Can you work these out from the model? Positions are in its coordinate system, mm. A direction names the side the tool comes from. Give positions to 0.01 mm unless a question says otherwise; leave off trailing zeros. Loops run counter-clockwise (first coordinate to the right, second up) from the corner with the lowest first, then second, coordinate; pieces in that order, holes last. Notation, with made-up numbers: (42, -35.75) - (65, -35.75) arc R24 ccw to (65, -15.75) - close; hole circle Ø6 at (38.5, -14). An arc over 180 degrees is marked (long way). Answer as a JSON object with one key per item and string values.
```python
from build123d import *

# Parameters (mm, degrees)
SKETCH1_W                                   = 304.8
SKETCH1_H                                   = 76.2
BOSS_EXTRUDE1_DEPTH                         = 6.35
SKETCH3_W                                   = 25.4
SKETCH3_H                                   = 50.8
CUT_EXTRUDE2_DEPTH                          = 25.4
BOSS_EXTRUDE2_DEPTH                         = 19.05
BOSS_EXTRUDE3_DEPTH                         = 304.8
BOSS_EXTRUDE4_DEPTH                         = 15.24
BOSS_EXTRUDE5_DEPTH                         = 15.24
CBORE_FOR_8_BINDING_HEAD_MACHINE_SC_2_COUNT = 2
CBORE_FOR_8_BINDING_HEAD_MACHINE_SC_2_PITCH = 238.76
CBORE_FOR_8_BINDING_HEAD_MACHINE_SC_3_COUNT = 2
CBORE_FOR_8_BINDING_HEAD_MACHINE_SC_3_PITCH = 255.670904094
CBORE_FOR_8_BINDING_HEAD_MACHINE_SC_4_COUNT = 2
CBORE_FOR_8_BINDING_HEAD_MACHINE_SC_4_PITCH = 91.44
SKETCH12_R                                  = 2.2479
CUT_EXTRUDE3_DEPTH                          = 23.0345001


with BuildPart() as part:
    # Sketch1 → Boss-Extrude1 (new body)
    with BuildSketch(Plane(origin=(0, 0, 0), x_dir=(1, 0, 0), z_dir=(0, 1, 0))):
        Rectangle(SKETCH1_W, SKETCH1_H)
    extrude(amount=-BOSS_EXTRUDE1_DEPTH)

    # Sketch3 → Cut-Extrude2 (cut)
    with BuildSketch(Plane(origin=(0, 0, 0), x_dir=(1, 0, 0), z_dir=(0, 1, 0))):
        with Locations((133.35, 0)):
            Rectangle(SKETCH3_W, SKETCH3_H)
    extrude(amount=-CUT_EXTRUDE2_DEPTH, mode=Mode.SUBTRACT)

    # Sketch4 → Boss-Extrude2 (add)
    with BuildSketch(Plane(origin=(0, 0, 0), x_dir=(1, 0, 0), z_dir=(0, 1, 0))):
        Polygon((152.4, 38.1), (-152.4, 38.1), (-152.4, 31.75), (146.05, 31.75), (152.4, 31.75), align=None)
        Polygon((146.05, -31.75), (-152.4, -31.75), (-152.4, -38.1), (152.4, -38.1), (152.4, -31.75), align=None)
        Polygon((152.4, -31.75), (152.4, 31.75), (146.05, 31.75), (146.05, 25.4), (146.05, -25.4), (146.05, -31.75), align=None)
    extrude(amount=BOSS_EXTRUDE2_DEPTH)

    # Sketch5 → Boss-Extrude3 (add)
    with BuildSketch(Plane.ZY.offset(152.4)):
        with BuildLine():
            Line((38.1, -6.35), (-38.1, -6.35))
            Line((-38.1, -6.35), (-38.1, -12.7))
            ThreePointArc((-38.1, -12.7), (0, -25.4), (38.1, -12.7))
            Line((38.1, -12.7), (38.1, -6.35))
        make_face()
    extrude(amount=-BOSS_EXTRUDE3_DEPTH)

    # Sketch8 → Boss-Extrude4 (add)
    with BuildSketch(Plane.ZY.offset(127)):
        with BuildLine():
            Line((-38.1, -12.7), (-38.1, 6.6675))
            Line((-38.1, 6.6675), (-53.34, 6.6675))
            Line((-53.34, 6.6675), (-53.34, 3.645763686))
            ThreePointArc((-53.34, 3.645763686), (-46.444745641, -5.202835962), (-38.1, -12.7))
        make_face()
        with BuildLine():
            Line((53.34, 3.645763686), (53.34, 6.6675))
            Line((53.34, 6.6675), (38.1, 6.6675))
            Line((38.1, 6.6675), (38.1, -12.7))
            ThreePointArc((38.1, -12.7), (46.444745641, -5.202835962), (53.34, 3.645763686))
        make_face()
    extrude(amount=-BOSS_EXTRUDE4_DEPTH)

    # Sketch9 → Boss-Extrude5 (add)
    with BuildSketch(Plane.ZY.offset(-111.76)):
        with BuildLine():
            Line((-38.1, -12.7), (-38.1, 6.6675))
            Line((-38.1, 6.6675), (-53.34, 6.6675))
            Line((-53.34, 6.6675), (-53.34, 3.645763686))
            ThreePointArc((-53.34, 3.645763686), (-46.444745641, -5.202835962), (-38.1, -12.7))
        make_face()
        with BuildLine():
            Line((53.34, 3.645763686), (53.34, 6.6675))
            Line((53.34, 6.6675), (38.1, 6.6675))
            Line((38.1, 6.6675), (38.1, -12.7))
            ThreePointArc((38.1, -12.7), (46.444745641, -5.202835962), (53.34, 3.645763686))
        make_face()
    extrude(amount=-BOSS_EXTRUDE5_DEPTH)

    # Sketch11 → CBORE for #8 Binding Head Machine Screw1 (revolve, cut)
    with BuildSketch(Plane(origin=(-119.38, -6.0325, -45.72), x_dir=(0, 0, -1), z_dir=(1, 0, 0))):
        Polygon((0, 0), (0, 25.0825), (2.2479, 25.0825), (2.2479, 2.667), (4.7625, 2.667), (4.7625, 0), align=None)
    cbore_for_8_binding_head_machine_screw1 = revolve(axis=Axis((-119.38, -12.3825, -45.72), (0, 1, 0)), mode=Mode.SUBTRACT)

    # CBORE for _8 Binding Head Machine Sc 2: CBORE for #8 Binding Head Machine Screw1 ×2
    with Locations(*[(i * CBORE_FOR_8_BINDING_HEAD_MACHINE_SC_2_PITCH, 0, 0) for i in range(1, CBORE_FOR_8_BINDING_HEAD_MACHINE_SC_2_COUNT)]):
        add(cbore_for_8_binding_head_machine_screw1, mode=Mode.SUBTRACT)

    # CBORE for _8 Binding Head Machine Sc 3: CBORE for #8 Binding Head Machine Screw1 ×2
    with Locations(*[Vector(0.933856752, 0, 0.357647267) * (i * CBORE_FOR_8_BINDING_HEAD_MACHINE_SC_3_PITCH) for i in range(1, CBORE_FOR_8_BINDING_HEAD_MACHINE_SC_3_COUNT)]):
        add(cbore_for_8_binding_head_machine_screw1, mode=Mode.SUBTRACT)

    # CBORE for _8 Binding Head Machine Sc 4: CBORE for #8 Binding Head Machine Screw1 ×2
    with Locations(*[(0, 0, i * CBORE_FOR_8_BINDING_HEAD_MACHINE_SC_4_PITCH) for i in range(1, CBORE_FOR_8_BINDING_HEAD_MACHINE_SC_4_COUNT)]):
        add(cbore_for_8_binding_head_machine_screw1, mode=Mode.SUBTRACT)

    # Sketch12 → Cut-Extrude3 (cut, through all)
    with BuildSketch(Plane.XZ.offset(3.3655)):
        with BuildLine():
            Line((-123.509642203, -48.092227124), (-115.250357797, -48.092227124))
            ThreePointArc((-115.250357797, -48.092227124), (-119.38, -40.9575), (-123.509642203, -48.092227124))
        make_face()
        with BuildLine():
            ThreePointArc((-114.6175, -45.72), (-120.607596281, -41.118433569), (-123.509642203, -48.092227124))
            Line((-123.509642203, -48.092227124), (-115.250357797, -48.092227124))
            ThreePointArc((-115.250357797, -48.092227124), (-114.778433569, -46.947596281), (-114.6175, -45.72))
        make_face()
        with BuildLine():
            Line((-115.250357797, -48.092227124), (-123.509642203, -48.092227124))
            ThreePointArc((-123.509642203, -48.092227124), (-119.38, -50.4825), (-115.250357797, -48.092227124))
        make_face()
        with BuildLine():
            Line((-123.509642203, 48.092227124), (-115.250357797, 48.092227124))
            ThreePointArc((-115.250357797, 48.092227124), (-119.38, 50.4825), (-123.509642203, 48.092227124))
        make_face()
        with BuildLine():
            ThreePointArc((-123.509642203, 48.092227124), (-119.38, 40.9575), (-115.250357797, 48.092227124))
            Line((-115.250357797, 48.092227124), (-123.509642203, 48.092227124))
        make_face()
        with Locations((-119.38, 45.72)):
            Circle(SKETCH12_R, mode=Mode.SUBTRACT)
        with BuildLine():
            ThreePointArc((124.1425, 45.72), (123.981566431, 46.947596281), (123.509642203, 48.092227124))
            Line((123.509642203, 48.092227124), (115.250357797, 48.092227124))
            ThreePointArc((115.250357797, 48.092227124), (118.152403719, 41.118433569), (124.1425, 45.72))
        make_face()
        with BuildLine():
            Line((115.250357797, 48.092227124), (123.509642203, 48.092227124))
            ThreePointArc((123.509642203, 48.092227124), (119.38, 50.4825), (115.250357797, 48.092227124))
        make_face()
        with BuildLine():
            Line((123.509642203, 48.092227124), (115.250357797, 48.092227124))
            ThreePointArc((115.250357797, 48.092227124), (119.38, 40.9575), (123.509642203, 48.092227124))
        make_face()
        with BuildLine():
            Line((115.250357797, -48.092227124), (123.509642203, -48.092227124))
            ThreePointArc((123.509642203, -48.092227124), (119.38, -40.9575), (115.250357797, -48.092227124))
        make_face()
        with BuildLine():
            ThreePointArc((124.1425, -45.72), (118.152403719, -41.118433569), (115.250357797, -48.092227124))
            Line((115.250357797, -48.092227124), (123.509642203, -48.092227124))
            ThreePointArc((123.509642203, -48.092227124), (123.981566431, -46.947596281), (124.1425, -45.72))
        make_face()
        with BuildLine():
            Line((123.509642203, -48.092227124), (115.250357797, -48.092227124))
            ThreePointArc((115.250357797, -48.092227124), (119.38, -50.4825), (123.509642203, -48.092227124))
        make_face()
        with Locations((-119.38, 45.72)):
            Circle(SKETCH12_R)
    extrude(amount=CUT_EXTRUDE3_DEPTH, mode=Mode.SUBTRACT)


solid = part.part
```
1) Imagine slicing it at A-A on x = -19. Write out the boundary of the cut face in (y, z).
Check sheet entries:
{"outline": "(-12.7, -38.1) - (19.05, -38.1) - (19.05, -31.75) - (0, -31.75) - (0, 31.75) - (19.05, 31.75) - (19.05, 38.1) - (-12.7, 38.1) arc R63.5 ccw to start"}
2) I need wall thicknesses on L1, parallel to X at y = 2.25, z = -45.72; L2, parallel to X at y = -5.3, z = 45.72; L3, parallel to Z at x = 46, y = 1. Which ranges of each line are inside material? Lowest first, please.
Check sheet entries:
{"L1": "-127 to -121.63, -117.13 to -111.76, 111.76 to 117.13, 121.63 to 127", "L2": "-127 to -124.14, -114.62 to -111.76, 111.76 to 114.62, 124.14 to 127", "L3": "-38.1 to -31.75, 31.75 to 38.1"}
3) Imagine slicing it at D-D on y = -16. Write out the boundary of the cut face in (x, z).
Check sheet entries:
{"outline": "(-152.4, -33.25) - (152.4, -33.25) - (152.4, 33.25) - (-152.4, 33.25) - close"}
4) Which directions (+Z, -Z, +X, -X, +Y, -Y) give clear straight access to the entire face, cutting with the end or side of a thin tool? Please do faces 4 (the flat face through (-5, 0, 0)), 5 (the flat face through (-119, -3.366, 43)), 6 (the flat face through (-127, -1, 44)), 7 (the flat face through (-111.76, -1, -44)).
Check sheet entries:
{"face 4": "-X, +Y", "face 5": "-Y", "face 6": "+Z, -X, +Y, -Y", "face 7": "-Z, +Y, -Y"}
5) If we mould it in two halves opening along Z, with no side actions, what happens to faces 1 (the flat face through (-2, 3, 38.1)), 2 (the flat face through (118, 6.668, 48)), 3 (the flat face through (133, -6.35, 0))? For each: released by +Z, released by -Z, zero draft, split by the parting line, or undercut.
Check sheet entries:
{"face 1": "released by +Z", "face 2": "zero draft", "face 3": "undercut"}
6) I'm going to push flat-ended pins straight in: P1, Ø2.5, axis at x = -119.38, z = -45.72, coming from the +Y side; P2, Ø7.5, axis at x = 121, z = 44, coming from the +Y side; P3, Ø5, axis at y = 1.5, z = 0, coming from the -X side; P4, Ø5.5, axis at x = -120.5, z = -44.5, coming from the -Y side. Where does each tip first touch, or does it pass through?
Check sheet entries:
{"P1": "through", "P2": "y = 6.67", "P3": "x = -152.4", "P4": "y = -3.37"}
7) Imagine slicing it at B-B on y = 13. Write out the boundary of the cut face in (x, z), and give its area (3 significant figures).
Check sheet entries:
{"outline": "(-152.4, -38.1) - (152.4, -38.1) - (152.4, 38.1) - (-152.4, 38.1) - (-152.4, 31.75) - (146.05, 31.75) - (146.05, -31.75) - (-152.4, -31.75) - close", "area": "4,270 mm2"}
8) Imagine slicing it at C-C on z = -28.5. Write out the boundary of the cut face in (x, y), and give its area (3 significant figures).
Check sheet entries:
{"outline": "(-152.4, -18.65) - (152.4, -18.65) - (152.4, 19.05) - (146.05, 19.05) - (146.05, 0) - (-152.4, 0) - close", "area": "5,800 mm2"}
